from build123d import *

# Parameters (mm, degrees)
BOSS_EXTRUDE1_DEPTH = 10
BOSS_EXTRUDE2_DEPTH = 15


with BuildPart() as part:
    # Sketch1 → Boss-Extrude1 (new body)
    with BuildSketch(Plane.XY):
        with BuildLine():
            Line((-30, 0), (0, 0))
            Line((0, 0), (0, 25))
            ThreePointArc((0, 25), (-19.52562419, 17.930749028), (-30, 0))
        make_face()
    extrude(amount=BOSS_EXTRUDE1_DEPTH)

    # Sketch2 → Boss-Extrude2 (add)
    with BuildSketch(Plane.XY.offset(10)):
        with BuildLine():
            Line((-30, 25), (0, 0))
            ThreePointArc((0, 0), (-10.47437581, 17.930749028), (-30, 25))
        make_face()
    extrude(amount=BOSS_EXTRUDE2_DEPTH)


solid = part.part
Here's how the part is built. I have some questions about the finished solid (model axes, mm). A direction names the side the tool comes from. Round coordinates to 2 decimals unless told otherwise and drop trailing zeros. Write each loop counter-clockwise with the first axis right and the second up, starting at its lowest first coordinate (ties: lowest second). Pieces come first, ordered by that corner, then holes. Notation, with made-up numbers: (-13, 2) -> (-5, 2) arc R6 cw to (-5, 7) -> close; hole circle Ø11 at (1.5, 65.25). An arc over 180 degrees is marked (long way). One line per item, written item: value.
1) Suppose I cut it at D-D on y = 10.25. List the corners of the cut face in (x, z) for me.
Filled sheet:
outline: (-26.12, 0) -> (0, 0) -> (0, 10) -> (-3.88, 10) -> (-3.88, 25) -> (-12.3, 25) -> (-12.3, 10) -> (-26.12, 10) -> close
2) Suppose I cut it at A-A on x = -24. List the corners of the cut face in (y, z) for me.
Filled sheet:
outline: (0, 0) -> (13.32, 0) -> (13.32, 10) -> (0, 10) -> close; (20, 10) -> (24.4, 10) -> (24.4, 25) -> (20, 25) -> close
3) Suppose I cut it at C-C on z = 12. List the corners of the cut face in (x, y) for me, plus the area to 3 significant figures.
Filled sheet:
outline: (-30, 25) -> (0, 0) arc R30.5 ccw to start
area: 189 mm2
4) I'm going to push flat-ended pins straight in: pin 1 Ø4 at (y, z) = (14, 13) entering from -X; pin 2 Ø10 at (x, z) = (-8, 19.5) entering from +Y; pin 3 Ø1.5 at (y, z) = (11.5, 14) entering from +X. Where does each tip first touch, or does it pass through?
Filled sheet:
pin 1: stops at x = -19.2
pin 2: stops at y = 19.82
pin 3: stops at x = -4.19
5) For faces 1 (the face through (-19, 7, 10)), 2 (the face through (-4, 18, 10)), 3 (the face through (-23, 22, 10)), which set-ups out of +Z, -Z, +X, -X, +Y, -Y let a thin tool reach every point of the face, with its end or its side?
Filled sheet:
face 1: +Z, -X, -Y
face 2: +Z, +X, +Y
face 3: -Z, -X, +Y
6) Suppose I cut it at B-B on y = 21.5. List the corners of the cut face in (x, z) for me, plus the area to 3 significant figures.
Filled sheet:
outline: (-25.8, 10) -> (-15.81, 10) -> (-15.81, 25) -> (-25.8, 25) -> close; (-14.19, 0) -> (0, 0) -> (0, 10) -> (-14.19, 10) -> close
area: 292 mm2
7) If I drill on line 1 (Z direction, x = -11, y = 21); line 2 (X direction, y = 22, z = 5.75); line 3 (X direction, y = 11, z = 20.5), over which ranges is the centre line in solid material (lowest first)? Write a range as [from, to].
Filled sheet:
line 1: z = [0, 10]
line 2: x = [-13.19, 0]
line 3: x = [-13.2, -4.35]
